For this review, use the dimensioned drawing (mm, ordinates from the lowest corner) and the shaded views. A direction names the side the tool comes from. Round coordinates to 2 decimals unless told otherwise and drop trailing zeros. Loops run counter-clockwise (first coordinate to the right, second up) from the corner with the lowest first, then second, coordinate; pieces in that order, holes last. Notation, with made-up numbers: (-13, -35) - (31, -35) arc R21 cw to (31, -24) - close; hole circle Ø10 at (-13.5, 5). An arc over 180 degrees is marked (long way). One line per question, with ' | ' between items. Start each with the question number.
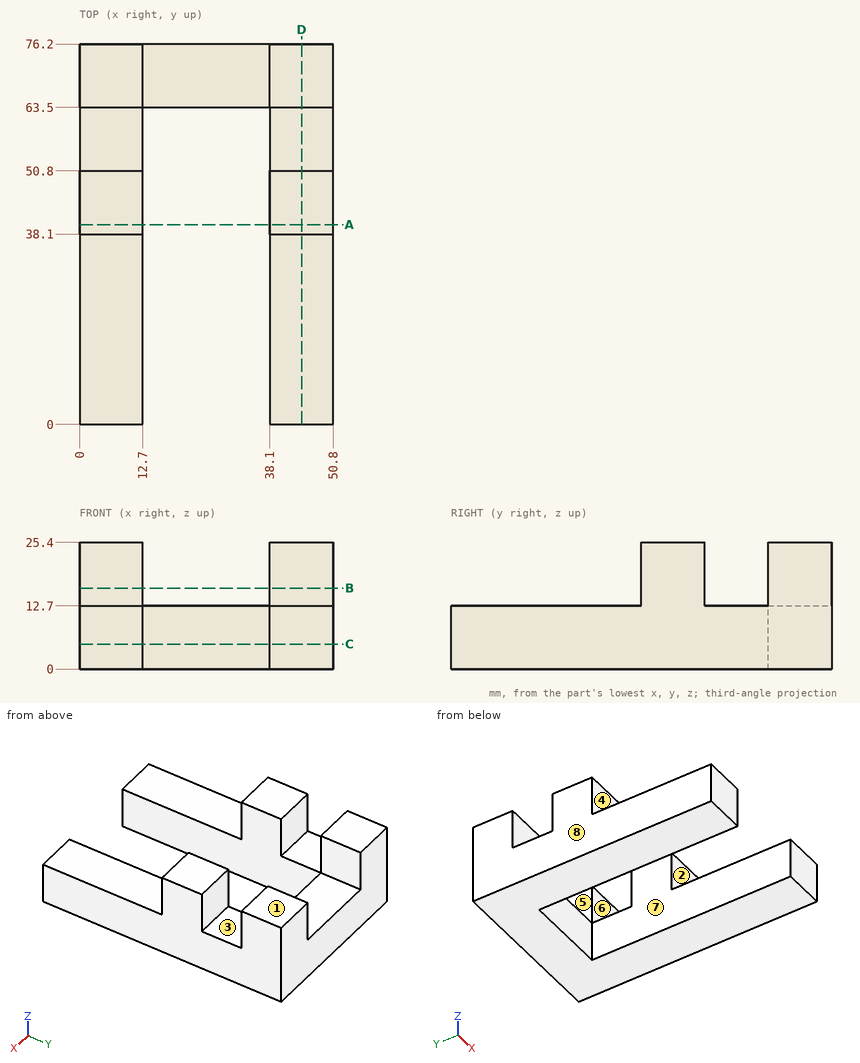
1. Clearance check with flat-ended pins moving along their axes: P1, Ø2, axis at x = 6.5, z = 21, coming from the -Y side; P2, Ø4, axis at x = 3.5, y = 16, coming from the +Z side; P3, Ø4, axis at x = 20, z = 5, coming from the -Y side. State where each tip first meets the part, or that it passes through.
2. Take a section at B-B, the plane z = 16.25. Give the boundary of the cut face in (x, y), then the cut area to 3 significant figures.
3. Take a section at D-D, the plane x = 44.5. Give the boundary of the cut face in (y, z).
4. Take a section at A-A, the plane y = 40. Give the boundary of the cut face in (x, z), then the cut area to 3 significant figures.
5. The part is to be moulded in two halves that separate along Y. For the marked faces 1, 2 and 3, say which applies: pulls with the +Y half, pulls with the -Y half, needs draft (parallel to the pull), parting line crosses it, or undercut.
6. Machinability: for the marked faces 4, 5, 6, 7 and 8, which of the approach directions +Z, -Z, +X, -X, +Y, -Y give a long, thin tool a straight path to every point of the face, cutting with its end or side? Answer none if there is none.
7. To check wall thickness, follow line 1 along Y through (x, z) = (5.5, 22.5); line 2 along X through (y, z) = (42.5, 16); line 3 along Y through (x, z) = (17, 10.5). State the ranges of each line that lie inside material, in increasing order.
8. Take a section at C-C, the plane z = 5. Give the boundary of the cut face in (x, y).
Answer list:
1) P1: stops at y = 38.1 | P2: stops at z = 12.7 | P3: stops at y = 63.5
2) outline: (0, 38.1) - (12.7, 38.1) - (12.7, 50.8) - (0, 50.8) - close; (0, 63.5) - (12.7, 63.5) - (12.7, 76.2) - (0, 76.2) - close; (38.1, 38.1) - (50.8, 38.1) - (50.8, 50.8) - (38.1, 50.8) - close; (38.1, 63.5) - (50.8, 63.5) - (50.8, 76.2) - (38.1, 76.2) - close | area: 645 mm²
3) outline: (0, 0) - (76.2, 0) - (76.2, 25.4) - (63.5, 25.4) - (63.5, 12.7) - (50.8, 12.7) - (50.8, 25.4) - (38.1, 25.4) - (38.1, 12.7) - (0, 12.7) - close
4) outline: (0, 0) - (12.7, 0) - (12.7, 25.4) - (0, 25.4) - close; (38.1, 0) - (50.8, 0) - (50.8, 25.4) - (38.1, 25.4) - close | area: 645 mm²
5) face 1: needs draft | face 2: pulls with the -Y half | face 3: undercut
6) face 4: +Z, +X, -X, -Y | face 5: +Z, +Y, -Y | face 6: +Z, +X, -X | face 7: +Z, -Z, -Y | face 8: +Z, -Z, -X, +Y, -Y
7) line 1: y = 38.1 to 50.8, 63.5 to 76.2 | line 2: x = 0 to 12.7, 38.1 to 50.8 | line 3: y = 63.5 to 76.2
8) outline: (0, 0) - (12.7, 0) - (12.7, 63.5) - (38.1, 63.5) - (38.1, 0) - (50.8, 0) - (50.8, 76.2) - (0, 76.2) - close
